For this review, take the finished solid that the model builds, in its own axes (mm). Give positions to 0.01 mm unless a question says otherwise; leave off trailing zeros. Loops run counter-clockwise (first coordinate to the right, second up) from the corner with the lowest first, then second, coordinate; pieces in that order, holes last. Notation, with made-up numbers: (62.25, 80) - (68.25, 80) arc R22 cw to (68.25, 95) - close; hole circle Ø11 at (-21.75, 8). An arc over 180 degrees is marked (long way). Answer as CSV lines item,"result".
from build123d import *

# Parameters (mm, degrees)
SKETCH2_W           = 76.2
SKETCH2_H           = 101.6
BOSS_EXTRUDE1_DEPTH = 4.7625
SKETCH3_R           = 3.175
CUT_EXTRUDE1_DEPTH  = 6.35
SKETCH3_4_R         = 3.175
SKETCH3_4_R_2       = 14.2875
SKETCH3_4_R_3       = 2.4892
CUT_EXTRUDE2_DEPTH  = 6.35


with BuildPart() as part:
    # Sketch2 → Boss-Extrude1 (new body)
    with BuildSketch(Plane(origin=(0, 0, 0), x_dir=(0, 0, -1), z_dir=(1, 0, 0))):
        Rectangle(SKETCH2_W, SKETCH2_H)
    extrude(amount=BOSS_EXTRUDE1_DEPTH)

    # Sketch3 → Cut-Extrude1 (cut)
    with BuildSketch(Plane(origin=(4.7625, 0, 0), x_dir=(0, 0, -1), z_dir=(1, 0, 0))):
        with Locations((30.2768, 42.9768)):
            Circle(SKETCH3_R)
    extrude(amount=-CUT_EXTRUDE1_DEPTH, mode=Mode.SUBTRACT)

    # Sketch3<4> → Cut-Extrude2 (cut)
    with BuildSketch(Plane(origin=(4.7625, 0, 0), x_dir=(0, 0, -1), z_dir=(1, 0, 0))):
        with Locations((30.2768, -44.5643)):
            Circle(SKETCH3_4_R)
        with Locations((30.2768, 42.9768)):
            Circle(SKETCH3_4_R)
        with Locations((-30.2768, 42.9768)):
            Circle(SKETCH3_4_R)
        with Locations((-30.2768, -44.5643)):
            Circle(SKETCH3_4_R)
        with Locations((18.9484, 0)):
            Circle(SKETCH3_4_R_2)
        with Locations((-5.1816, -25.4)):
            Circle(SKETCH3_4_R_3)
        with Locations((0, -44.5643)):
            Circle(SKETCH3_4_R)
    extrude(amount=-CUT_EXTRUDE2_DEPTH, mode=Mode.SUBTRACT)


solid = part.part
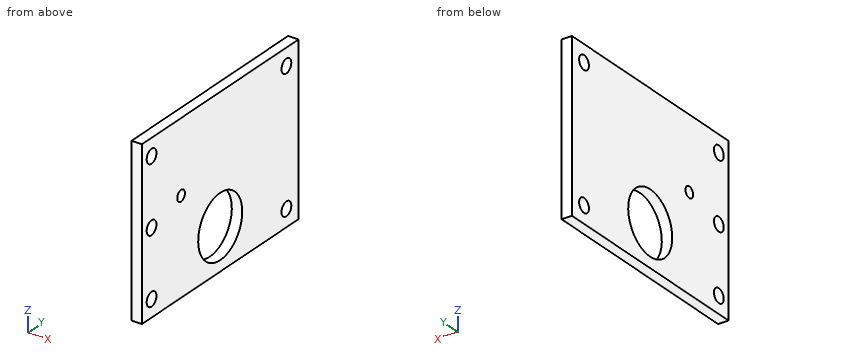
1) Insertion check: P1, Ø3, axis at y = -25.4, z = 5.18, coming from the +X side. The pin has a flat end and moves straight along its axis. Give the tip position at first contact, or say it passes through.
From the geometry:
P1,"passes through"
2) Wall thickness on line 1 (Y direction, x = 1.3, z = 0); line 2 (Z direction, x = 4.35, y = -43); line 3 (Y direction, x = 0.45, z = 32): over which ranges is each line inside the solid? List them lowest first. Write a range as from..to.
From the geometry:
line 1,"y = -50.8..-47.74, -41.39..50.8"
line 2,"z = -38.1..-33.04, -27.51..-2.76, 2.76..27.51, 33.04..38.1"
line 3,"y = -50.8..-47.23, -41.9..40.31, 45.64..50.8"
3) Consider section C-C on x = 1.6. Count the separate pieces of the cut face and the enclosed holes in it, and give its area (3 significant figures).
From the geometry:
separate pieces,"1"
enclosed holes,"7"
area,"6,920 mm^2"
4) Consider section B-B on y = -25.4. Write out the cut boundary in (x, z).
From the geometry:
outline,"(0, -38.1) - (4.76, -38.1) - (4.76, 2.69) - (0, 2.69) - close; (0, 7.67) - (4.76, 7.67) - (4.76, 38.1) - (0, 38.1) - close"
5) Consider section A-A on z = 0. Write out the cut boundary in (x, y), and give its area (3 significant figures).
From the geometry:
outline,"(0, -50.8) - (4.76, -50.8) - (4.76, -47.74) - (0, -47.74) - close; (0, -41.39) - (4.76, -41.39) - (4.76, 50.8) - (0, 50.8) - close"
area,"454 mm^2"
